```python
from build123d import *

# Parameters (mm, degrees)
SKETCH1_W           = 60
SKETCH1_H           = 30
BOSS_EXTRUDE1_DEPTH = 36.57
CUT_EXTRUDE1_DEPTH  = 60
CUT_EXTRUDE2_REACH  = 82.464
CUT_EXTRUDE3_DEPTH  = 73.14
SKETCH5_R           = 3.75
CUT_EXTRUDE4_DEPTH  = 30
SKETCH6_R           = 7.5
CUT_EXTRUDE5_DEPTH  = 20
SKETCH8_R           = 85
BOSS_EXTRUDE3_DEPTH = 31.6
CUT_EXTRUDE6_START  = -31.6
SKETCH9_R           = 7.5
CUT_EXTRUDE6_DEPTH  = 31.6
SKETCH11_W          = 40.5
SKETCH11_H          = 20.15
CUT_EXTRUDE7_DEPTH  = 26.6
BOSS_EXTRUDE4_DEPTH = 73.14
SKETCH13_R          = 7.5
CUT_EXTRUDE8_DEPTH  = 51.6
FILLET1_R           = 8
SKETCH14_W          = 14
SKETCH14_H          = 10
CUT_EXTRUDE9_DEPTH  = 84


with BuildPart() as part:
    # Sketch1 → Boss-Extrude1 (new, symmetric)
    with BuildSketch(Plane.XY):
        Rectangle(SKETCH1_W, SKETCH1_H)
    extrude(amount=BOSS_EXTRUDE1_DEPTH, both=True)

    # Sketch2 → Cut-Extrude1 (cut)
    with BuildSketch(Plane(origin=(30, 0, 0), x_dir=(0, 0, -1), z_dir=(1, 0, 0))):
        with BuildLine():
            ThreePointArc((6, -15), (0, -9), (-6, -15))
            Line((-6, -15), (6, -15))
        make_face()
    extrude(amount=-CUT_EXTRUDE1_DEPTH, mode=Mode.SUBTRACT)

    # Cut-Extrude2: up to this face of the body (flat: up to its plane)
    cut_extrude2_end = Plane(part.part.faces().sort_by_distance((0, 0, -36.57))[0])
    # Sketch3 → Cut-Extrude2 (cut, up to the picked face)
    with BuildSketch(Plane.XY.offset(36.57), mode=Mode.PRIVATE) as cut_extrude2_sk1:
        with BuildLine():
            Line((6.075, 0), (11.075, 0))
            Line((11.075, 0), (15.094237886, -15))
            Line((15.094237886, -15), (-15.094237886, -15))
            Line((-15.094237886, -15), (-11.075, 0))
            Line((-11.075, 0), (-6.075, 0))
            ThreePointArc((-6.075, 0), (0, 6.075), (6.075, 0))
        make_face()
    cut_extrude2_tool1 = split(extrude(cut_extrude2_sk1.sketch, amount=-CUT_EXTRUDE2_REACH, mode=Mode.PRIVATE), bisect_by=cut_extrude2_end, keep=Keep.BOTH, mode=Mode.PRIVATE)
    add(cut_extrude2_tool1.solids().sort_by(Axis((0, -6.537689, 36.57), (0, 0, -1)))[0], mode=Mode.SUBTRACT)

    # Sketch4 → Cut-Extrude3 (cut)
    with BuildSketch(Plane.XY.offset(36.57)):
        Polygon((30, 15), (30, -5), (10, 15), align=None)
        Polygon((-30, 15), (-30, -5), (-10, 15), align=None)
    extrude(amount=-CUT_EXTRUDE3_DEPTH, mode=Mode.SUBTRACT)

    # Sketch5 → Cut-Extrude4 (cut)
    with BuildSketch(Plane(origin=(0, 15, 0), x_dir=(1, 0, 0), z_dir=(0, 1, 0))):
        with Locations(Location((22, -26.57, 0), (0, 0, 180))):
            Circle(SKETCH5_R)
        with Locations(Location((-22, -26.57, 0), (0, 0, 180))):
            Circle(SKETCH5_R)
        with Locations(Location((22, 26.57, 0), (0, 0, 180))):
            Circle(SKETCH5_R)
        with Locations(Location((-22, 26.57, 0), (0, 0, 180))):
            Circle(SKETCH5_R)
    extrude(amount=-CUT_EXTRUDE4_DEPTH, mode=Mode.SUBTRACT)

    # Sketch6 → Cut-Extrude5 (cut)
    with BuildSketch(Plane(origin=(0, 15, 0), x_dir=(1, 0, 0), z_dir=(0, 1, 0))):
        with Locations(Location((22, -26.57, 0), (0, 0, 180))):
            Circle(SKETCH6_R)
        with Locations((-22, -26.57)):
            Circle(SKETCH6_R)
        with Locations(Location((22, 26.57, 0), (0, 0, 180))):
            Circle(SKETCH6_R)
        with Locations(Location((-22, 26.57, 0), (0, 0, 180))):
            Circle(SKETCH6_R)
    extrude(amount=-CUT_EXTRUDE5_DEPTH, mode=Mode.SUBTRACT)

    # Sketch8 → Boss-Extrude3 (add)
    with BuildSketch(Plane(origin=(0, 15, 0), x_dir=(1, 0, 0), z_dir=(0, 1, 0))):
        with Locations(Location((0, 0, 0), (0, 0, 180))):
            Circle(SKETCH8_R)
    extrude(amount=BOSS_EXTRUDE3_DEPTH)

    # Sketch9 → Cut-Extrude6 (cut)
    with BuildSketch(Plane.XZ.offset(-15).offset(CUT_EXTRUDE6_START)):
        with Locations(Location((22, 26.57, 0), (0, 0, 180))):
            Circle(SKETCH9_R)
        with Locations(Location((22, -26.57, 0), (0, 0, 180))):
            Circle(SKETCH9_R)
        with Locations(Location((-22, -26.57, 0), (0, 0, 180))):
            Circle(SKETCH9_R)
        with Locations((-22, 26.57)):
            Circle(SKETCH9_R)
    extrude(amount=CUT_EXTRUDE6_DEPTH, mode=Mode.SUBTRACT)

    # Sketch11 → Cut-Extrude7 (cut)
    with BuildSketch(Plane(origin=(0, 46.6, 0), x_dir=(1, 0, 0), z_dir=(0, 1, 0))):
        with Locations((-10.25, -0.075)):
            Rectangle(SKETCH11_W, SKETCH11_H)
    extrude(amount=-CUT_EXTRUDE7_DEPTH, mode=Mode.SUBTRACT)

    # Sketch12 → Boss-Extrude4 (add)
    with BuildSketch(Plane.XY.offset(36.57)):
        Polygon((30, -5), (30, 15), (10, 15), align=None)
        Polygon((-10, 15), (-30, -5), (-30, 15), align=None)
    extrude(amount=-BOSS_EXTRUDE4_DEPTH)

    # Sketch13 → Cut-Extrude8 (cut)
    with BuildSketch(Plane(origin=(0, 46.6, 0), x_dir=(1, 0, 0), z_dir=(0, 1, 0))):
        with Locations(Location((22, 26.57, 0), (0, 0, 180))):
            Circle(SKETCH13_R)
        with Locations(Location((-22, 26.57, 0), (0, 0, 180))):
            Circle(SKETCH13_R)
        with Locations(Location((-22, -26.57, 0), (0, 0, 180))):
            Circle(SKETCH13_R)
        with Locations(Location((22, -26.57, 0), (0, 0, 180))):
            Circle(SKETCH13_R)
    extrude(amount=-CUT_EXTRUDE8_DEPTH, mode=Mode.SUBTRACT)

    # Fillet1
    fillet1_edges = [part.edges().sort_by_distance(p)[0] for p in [
        (30, 15, 0),
        (-30, 15, 0),
        (0, 15, -36.57),
        (0, 15, 36.57),
    ]]
    fillet(fillet1_edges, radius=FILLET1_R)

    # Sketch14 → Cut-Extrude9 (cut)
    with BuildSketch(Plane.ZY.offset(-10)):
        with Locations((0.075, 25)):
            Rectangle(SKETCH14_W, SKETCH14_H)
    extrude(amount=-CUT_EXTRUDE9_DEPTH, mode=Mode.SUBTRACT)


solid = part.part
```
Verification items for the finished model (mm, model axes). A direction names the side the tool comes from. Coordinates: 2 decimals unless noted, no trailing zeros. Loops run counter-clockwise (first coordinate to the right, second up) from the corner with the lowest first, then second, coordinate; pieces in that order, holes last. Notation, with made-up numbers: (-35, 49.25) -> (-16, 49.25) arc R32 ccw to (-16, 78.25) -> close; hole circle Ø4 at (70, 2). An arc over 180 degrees is marked (long way). Put each result on its own line as item: value.
1. Tool access check on faces 5 (the face through (13.056, -7.395, 0.512)), 6 (the face through (30, -4, 1)), 7 (the face through (10, 36, 0)). Record the directions out of +Z, -Z, +X, -X, +Y, -Y that give a thin tool (end or side, any length) a straight path to the whole face; none if there is none.
Result set:
face 5: +Z, -Z, -Y
face 6: +Z, -Z, +X, -Y
face 7: +Y
2. Mould release check, pull along Z, two halves, no side actions. Record for faces 1 (the face through (-81.075, 30.579, 25.532)), 2 (the face through (-7, 1, 36.57)), 3 (the face through (-30.5, 33, 0)), 4 (the face through (18.423, -9.93, 27.696)): pulls with the +Z half, pulls with the -Z half, needs draft (parallel to the pull), parting line crosses it, or undercut.
Result set:
face 1: parting line crosses it
face 2: pulls with the +Z half
face 3: undercut
face 4: undercut
3. Section check D-D, the plane x = 0. Record the boundary of the cut face in (y, z) (3 decimals).
Result set:
outline: (6.075, -36.57) -> (7, -36.57) arc R8 cw to (15, -44.57) -> (15, -85) -> (46.6, -85) -> (46.6, -10) -> (20, -10) -> (20, 10.15) -> (46.6, 10.15) -> (46.6, 85) -> (15, 85) -> (15, 44.57) arc R8 cw to (7, 36.57) -> (6.075, 36.57) -> close
4. Gauge pin test, flat ends, axial feed: P1, Ø1.5, axis at y = 12.5, z = -48, coming from the -X side; P2, Ø1.5, axis at x = -8, z = 14, coming from the -Y side; P3, Ø6.5, axis at x = 14, y = -5.5, coming from the -Z side; P4, Ø24, axis at x = 3.5, y = -6, coming from the +Z side. Record the tip position at first contact, or that the pin passes through.
Result set:
P1: passes through
P2: stops at y = 0
P3: stops at z = -36.57
P4: stops at z = 36.57
5. Section check C-C, the plane z = 0. Record the boundary of the cut face in (x, y) (3 decimals), then the cut area to 3 significant figures.
Result set:
outline: (-85, 15) -> (-38, 15) arc R8 cw to (-30, 7) -> (-30, -9) -> (-13.487, -9) -> (-11.075, 0) -> (-6.075, 0) arc R6.075 cw to (6.075, 0) -> (11.075, 0) -> (13.487, -9) -> (30, -9) -> (30, 7) arc R8 cw to (38, 15) -> (85, 15) -> (85, 20) -> (-30.5, 20) -> (-30.5, 46.6) -> (-85, 46.6) -> close; (10, 30) -> (85, 30) -> (85, 46.6) -> (10, 46.6) -> close
area: 4,730 mm^2
6. Section check B-B, the plane x = -22. Give the number of separate pieces and of enclosed holes in the cut face, then the cut area to 3 significant figures.
Result set:
separate pieces: 3
enclosed holes: 0
area: 5,120 mm^2
7. Thickness scan on line 1 (X direction, y = 1, z = -26); line 2 (Z direction, x = -22, y = 3); line 3 (X direction, y = 18, z = 26). Record the ranges inside material, lowest first.
Result set:
line 1: x = -30 to -29.48, -14.52 to -5.99, 5.99 to 14.52, 29.48 to 30
line 2: z = -36.57 to -34.07, -19.07 to 19.07, 34.07 to 36.57
line 3: x = -80.93 to -29.48, -14.52 to 14.52, 29.48 to 80.93
8. Section check A-A, the plane y = 3.5. Record the boundary of the cut face in (x, z).
Result set:
outline: (-30, -36.57) -> (-4.97, -36.57) -> (-4.97, 36.57) -> (-30, 36.57) -> close; (4.97, -36.57) -> (30, -36.57) -> (30, 36.57) -> (4.97, 36.57) -> close; hole circle Ø15 at (-22, -26.57); hole circle Ø15 at (-22, 26.57); hole circle Ø15 at (22, -26.57); hole circle Ø15 at (22, 26.57)
